For this review, take the finished solid that the model builds, in its own axes (mm). Give positions to 0.01 mm unless a question says otherwise; leave off trailing zeros. Write each loop counter-clockwise with the first axis right and the second up, starting at its lowest first coordinate (ties: lowest second). Pieces come first, ordered by that corner, then holes.
Q1. For line 1 (Z direction, x = 2.8, y = -1); line 2 (Y direction, x = 2, z = 0); line 3 (Z direction, x = 1, y = -86), list the stretches that pass through material, from the lowest coordinate up.
Q2. We need section A-A (y = -218.5). Write out the cut boundary in (x, z) (3 decimals), then the cut area to 3 significant figures.
Q3. We need section B-B (x = 1.3). Give the number of separate pieces and of enclosed holes in the cut face, then the cut area to 3 significant figures.
Q4. We need section C-C (z = 211). Write out the cut boundary in (x, y) (3 decimals).
Q5. Insertion check: P1, Ø0.5, axis at x = 1.5, z = -25, coming from the -Y side; P2, Ø5.5, axis at y = -39.28, z = 223.55, coming from the +X side; P3, Ø1.6, axis at x = 1.5, y = -178, coming from the +Z side; P4, Ø1.5, axis at x = 0.5, y = -46.5, coming from the +Z side. Each pin has a flat end and moves straight along its axis. Give the tip position at first contact, or say it passes through.
```python
from build123d import *

# Parameters (mm, degrees)
BOSS_EXTRUDE2_DEPTH = 3.175
SKETCH11_W          = 25.4
SKETCH11_H          = 25.436159883
BOSS_EXTRUDE4_DEPTH = 3.175
SKETCH12_R          = 3.175
BOSS_EXTRUDE5_DEPTH = 3.175
SKETCH13_R          = 3.175
BOSS_EXTRUDE6_DEPTH = 3.175
SKETCH14_R          = 14.2875
BOSS_EXTRUDE7_DEPTH = 3.175
SKETCH15_R          = 3.175
SKETCH15_R_2        = 2.54
CUT_EXTRUDE1_DEPTH  = 4.175


with BuildPart() as part:
    # Sketch9 → Boss-Extrude2 (new body)
    with BuildSketch(Plane(origin=(0, 0, 0), x_dir=(0, 0, -1), z_dir=(1, 0, 0))):
        with BuildLine():
            Line((0, -126.954378983), (0, -152.390538866))
            ThreePointArc((0, -152.390538866), (-140.790499807, -58.317334473), (-107.756383421, 107.756383421))
            Line((-107.756383421, 107.756383421), (-89.795871179, 125.716895663))
            Line((-89.795871179, 125.716895663), (-71.809790038, 107.730814523))
            Line((-71.809790038, 107.730814523), (-89.770302281, 89.770302281))
            ThreePointArc((-89.770302281, 89.770302281), (-117.290552306, -48.583337503), (0, -126.954378983))
        make_face()
    extrude(amount=BOSS_EXTRUDE2_DEPTH)

    # Sketch11 → Boss-Extrude4 (add)
    with BuildSketch(Plane(origin=(0, 0, 0), x_dir=(0, 0, -1), z_dir=(1, 0, 0))):
        with Locations((12.7, -139.672458925)):
            Rectangle(SKETCH11_W, SKETCH11_H)
    extrude(amount=BOSS_EXTRUDE4_DEPTH)

    # Sketch12 → Boss-Extrude5 (add)
    with BuildSketch(Plane(origin=(0, 0, 0), x_dir=(0, 0, -1), z_dir=(1, 0, 0))):
        with BuildLine():
            ThreePointArc((-1.596710848, -228.181271676), (11.103289152, -240.881271676), (23.803289152, -228.181271676))
            Line((23.803289152, -228.181271676), (23.803289152, -152.390538866))
            Line((23.803289152, -152.390538866), (0, -152.390538866))
            ThreePointArc((0, -152.390538866), (-0.79836638, -152.388447551), (-1.596710848, -152.382173664))
            Line((-1.596710848, -152.382173664), (-1.596710848, -228.181271676))
        make_face()
        with Locations((11.103289152, -228.181271676)):
            Circle(SKETCH12_R, mode=Mode.SUBTRACT)
    extrude(amount=BOSS_EXTRUDE5_DEPTH)

    # Sketch13 → Boss-Extrude6 (add)
    with BuildSketch(Plane(origin=(0, 0, 0), x_dir=(0, 0, -1), z_dir=(1, 0, 0))):
        with BuildLine():
            Line((-175.921744047, -157.217647079), (-117.615441364, -113.032446562))
            ThreePointArc((-117.615441364, -113.032446562), (-109.43511183, -110.464604073), (-101.487144145, -113.680411283))
            ThreePointArc((-101.487144145, -113.680411283), (-121.45550521, -92.040407377), (-136.889329567, -66.964078331))
            ThreePointArc((-136.889329567, -66.964078331), (-135.942652679, -75.485545881), (-140.626971786, -82.666685125))
            Line((-140.626971786, -82.666685125), (-160.306949591, -97.58040329))
            ThreePointArc((-160.306949591, -97.58040329), (-171.19425961, -99.744336405), (-179.624122676, -92.522595986))
            Line((-179.624122676, -92.522595986), (-190.009209059, -68.638532465))
            ThreePointArc((-190.009209059, -68.638532465), (-189.548026602, -57.559851452), (-180.560256724, -51.066019389))
            Line((-180.560256724, -51.066019389), (-156.267984197, -46.797896728))
            ThreePointArc((-156.267984197, -46.797896728), (-147.818260582, -48.251780205), (-142.218034883, -54.744012368))
            ThreePointArc((-142.218034883, -54.744012368), (-150.091480412, -26.370890083), (-152.361266177, 2.986788389))
            ThreePointArc((-152.361266177, 2.986788389), (-155.413049284, -5.02559117), (-162.861116025, -9.272697026))
            Line((-162.861116025, -9.272697026), (-234.783717211, -21.90941035))
            ThreePointArc((-234.783717211, -21.90941035), (-243.771487088, -28.403242413), (-244.232669546, -39.481923426))
            Line((-244.232669546, -39.481923426), (-195.238917132, -152.159839775))
            ThreePointArc((-195.238917132, -152.159839775), (-186.809054067, -159.381580194), (-175.921744047, -157.217647079))
        make_face()
        with Locations((-180.989788445, -137.156185968)):
            Circle(SKETCH13_R, mode=Mode.SUBTRACT)
        with Locations((-223.548763187, -39.27724509)):
            Circle(SKETCH13_R, mode=Mode.SUBTRACT)
    extrude(amount=BOSS_EXTRUDE6_DEPTH)

    # Sketch14 → Boss-Extrude7 (add)
    with BuildSketch(Plane(origin=(0, 0, 0), x_dir=(0, 0, -1), z_dir=(1, 0, 0))):
        with BuildLine():
            Line((-29.799778624, 38.874174032), (-100.328890576, 92.993065071))
            Line((-100.328890576, 92.993065071), (-115.791430873, 72.841890227))
            Line((-115.791430873, 72.841890227), (-45.262318921, 18.722999189))
            ThreePointArc((-45.262318921, 18.722999189), (-48.592985775, 6.160352763), (-48.502549248, -6.836002425))
            Line((-48.502549248, -6.836002425), (-121.562281943, -36.60636491))
            ThreePointArc((-121.562281943, -36.60636491), (-117.290552306, -48.583337503), (-111.842122761, -60.072905036))
            Line((-111.842122761, -60.072905036), (-39.130265149, -29.462697807))
            ThreePointArc((-39.130265149, -29.462697807), (-27.212895153, -40.726975705), (-12.2454793, -47.426537396))
            Line((-12.2454793, -47.426537396), (-12.7, -126.317553583))
            ThreePointArc((-12.7, -126.317553583), (-6.357978189, -126.795072682), (0, -126.954378983))
            Line((0, -126.954378983), (12.2454793, -126.954378983))
            Line((12.2454793, -126.954378983), (12.2454793, -47.426537396))
            ThreePointArc((12.2454793, -47.426537396), (44.033981815, 21.453127004), (-29.799778624, 38.874174032))
        make_face()
        Circle(SKETCH14_R, mode=Mode.SUBTRACT)
    extrude(amount=BOSS_EXTRUDE7_DEPTH)

    # Sketch15 → Cut-Extrude1 (cut, through all)
    with BuildSketch(Plane(origin=(3.175, 0, 0), x_dir=(0, 0, -1), z_dir=(1, 0, 0))):
        with Locations((11.103289152, -228.181271676)):
            Circle(SKETCH15_R)
        with Locations((0, -55.741886393)):
            Circle(SKETCH15_R_2)
        with Locations((0, -97.196272786)):
            Circle(SKETCH15_R_2)
    extrude(amount=-CUT_EXTRUDE1_DEPTH, mode=Mode.SUBTRACT)


solid = part.part
```
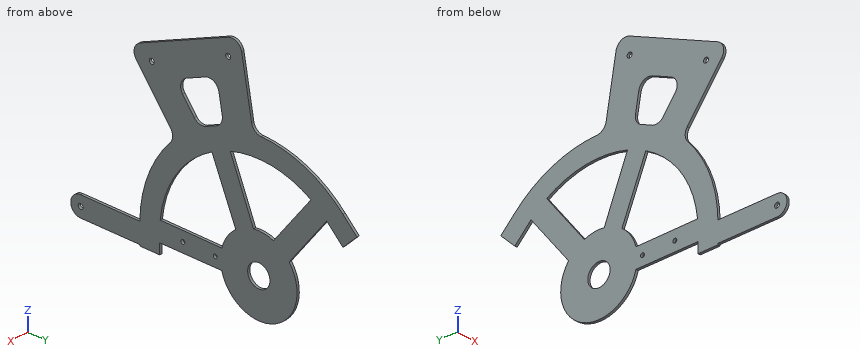
Computed:
1. line 1: z = -48.97 to -14.25, 14.25 to 48.97, 126.95 to 153.09
1. line 2: y = -234.35 to -99.74, -94.66 to -58.28, -53.2 to -14.29, 14.29 to 48.98
1. line 3: z = -12.25 to 12.47, 93.39 to 145.03, 182.46 to 224.01
2. outline: (0, -23.803) - (3.175, -23.803) - (3.175, 1.597) - (0, 1.597) - close
2. area: 80.6 mm2
3. separate pieces: 1
3. enclosed holes: 9
3. area: 34,400 mm2
4. outline: (0, -115.912) - (3.175, -115.912) - (3.175, -17.731) - (0, -17.731) - close
5. P1: stops at y = -152.39
5. P2: passes through
5. P3: stops at z = 1.6
5. P4: stops at z = 241.51
